Model file for the job. Use its own axes, mm. Face numbers are marked on the shaded views. Coordinates: 2 decimals unless noted, no trailing zeros. Write each loop counter-clockwise with the first axis right and the second up, starting at its lowest first coordinate (ties: lowest second). Pieces come first, ordered by that corner, then holes. Notation, with made-up numbers: M 59.25,26.5 L 116.25,26.5 A26 ccw 116.25,53.5 Z; hole C -32,9 d8. An arc over 180 degrees is marked long. One line per question, with ' | ' between items. Start each with the question number.
(1) Two-plate mould, pull along Y, no slides. Class the marked faces 1, 2 and 3: +Y half, -Y half, draft (parallel to the pull), parting line (faces both ways), or undercut.
(2) Cut at B-B (z = 36.5). Write the cut outline in (x, y), plus the area to 3 significant figures.
(3) Flat gauge pins, fed straight in: pin 1 Ø10 at (y, z) = (11, 58) entering from -X; pin 2 Ø8 at (x, z) = (12.5, 20.5) entering from -Y; pin 3 Ø3 at (x, z) = (-2.5, 63.5) entering from +Y. Where does each tip first touch, or does it go through?
(4) Cut at A-A (x = 0). Write the cut outline in (y, z), plus the area to 3 significant figures.
(5) Wall check: probe 1 along Y at (x, z) = (0, 63.5); probe 2 along Y at (x, z) = (-9, 50); probe 3 along Z at (x, y) = (8.5, -19.5). Give the ranges that are in metal, low to high.
(6) Cut at D-D (z = 14). Write the cut outline in (x, y).
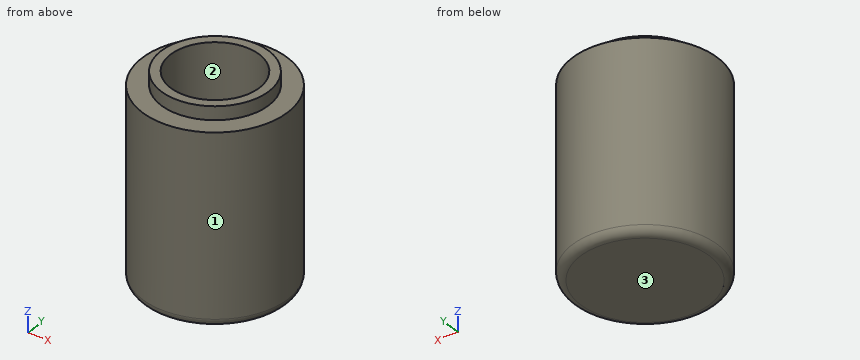
Solid Edge part; units mm, degrees
sketch "Sketch1" plane through (0, 0, 0) normal (0, 0, 1) x (1, 0, 0)
  circle A0 centre (0, 0) radius 27
extrude "Protrusion1" add sketch "Sketch1" along normal blind 70
sketch "Sketch2" plane through (0, 0, 70) normal (0, 0, 1) x (1, 0, 0)
  circle A0 centre (0, 0) radius 20
extrude "ProtrusiónExtruida_2" add sketch "Sketch2" along normal blind 5
hole "Agujero_1" at (0, 0, 75) direction (0, 0, -1) diameter 33 depth 41
fillet "Redondeo_1" radius 3 1 edges at (-27, 0, 0)
Filled in:
1) face 1: parting line | face 2: undercut | face 3: draft
2) outline: C 0,0 d54; hole C 0,0 d33 | area: 1,430 mm²
3) pin 1: x = -26.32 | pin 2: y = -25.63 | pin 3: y = 26.98
4) outline: M -27,3 A3 ccw -24,0 L 24,0 A3 ccw 27,3 L 27,70 L 20,70 L 20,75 L 16.5,75 L 16.5,34 L -16.5,34 L -16.5,75 L -20,75 L -20,70 L -27,70 Z | area: 2,620 mm²
5) probe 1: -27 to -16.5, 16.5 to 27 | probe 2: -25.46 to -13.83, 13.83 to 25.46 | probe 3: 0 to 70
6) outline: C 0,0 d54
